Could you check a few things on this drawing? It's one solid part, dimensions in mm from its lowest x, y, z. A direction names the side the tool comes from. Round coordinates to 2 decimals unless told otherwise and drop trailing zeros. Loops run counter-clockwise (first coordinate to the right, second up) from the corner with the lowest first, then second, coordinate; pieces in that order, holes last. Notation, with made-up numbers: M 1,0 L 15,0 A8 ccw 15,7 Z; hole C -0.5,53.25 d1. An arc over 180 degrees is marked long. Return JSON: item names as keys, results as strings.
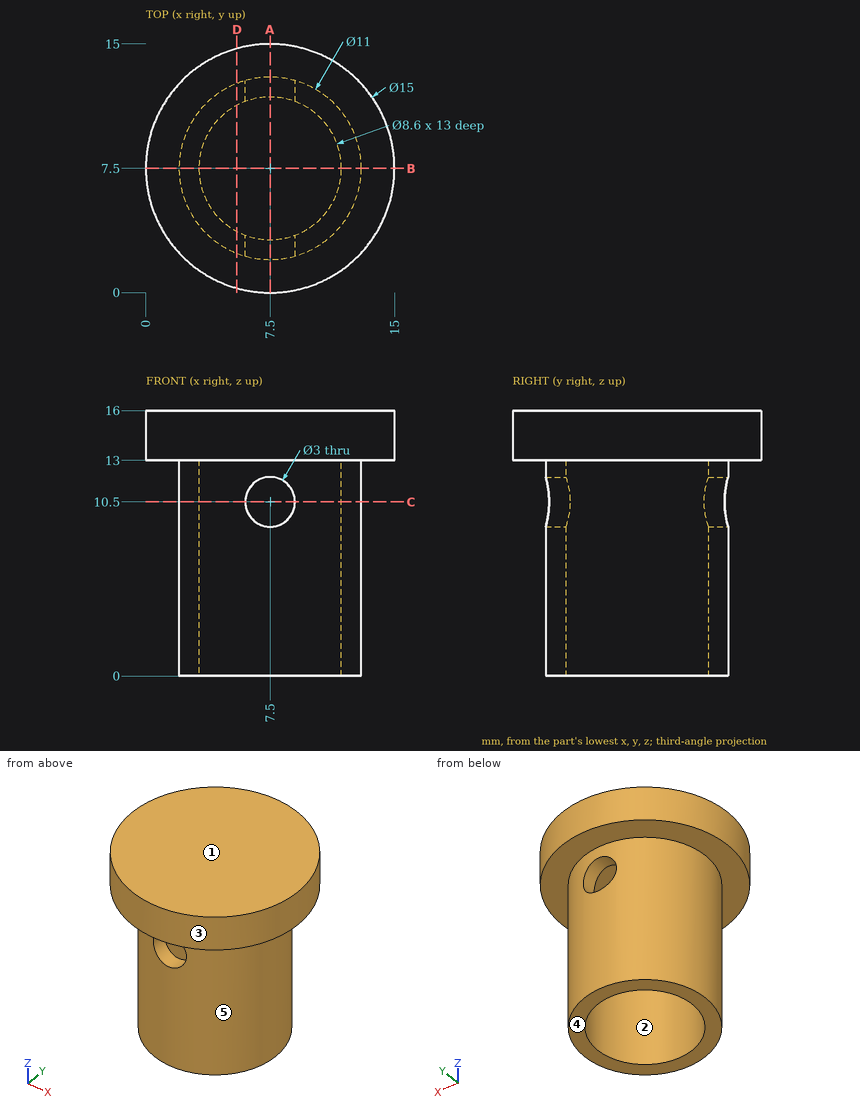
Q1. Suppose I cut it at C-C, the plane z = 10.5. Please give me the cut outline in (x, y), plus the area to 3 significant figures.
Results:
{"outline": "M 6,2.21 L 6,3.47 A4.3 cw 6,11.53 L 6,12.79 A5.5 ccw Z; M 9,2.21 A5.5 ccw 9,12.79 L 9,11.53 A4.3 cw 9,3.47 Z", "area": "29.6 mm2"}
Q2. Suppose I cut it at B-B, the plane y = 7.5. Please give me the cut outline in (x, z).
Results:
{"outline": "M 0,13 L 2,13 L 2,0 L 3.2,0 L 3.2,13 L 11.8,13 L 11.8,0 L 13,0 L 13,13 L 15,13 L 15,16 L 0,16 Z"}
Q3. Suppose I cut it at A-A, the plane x = 7.5. Please give me the cut outline in (y, z), plus the area to 3 significant figures.
Results:
{"outline": "M 0,13 L 2,13 L 2,12 L 3.2,12 L 3.2,13 L 11.8,13 L 11.8,12 L 13,12 L 13,13 L 15,13 L 15,16 L 0,16 Z; M 2,0 L 3.2,0 L 3.2,9 L 2,9 Z; M 11.8,0 L 13,0 L 13,9 L 11.8,9 Z", "area": "69.0 mm2"}
Q4. I'm going to push flat-ended pins straight in: pin 1 Ø4 at (x, z) = (7.5, 10.5) entering from +Y; pin 2 Ø3 at (x, z) = (11.5, 4.5) entering from -Y; pin 3 Ø3 at (y, z) = (11, 8) entering from -X. Where does each tip first touch, or does it pass through?
Results:
{"pin 1": "stops at y = 13", "pin 2": "stops at y = 2.6", "pin 3": "stops at x = 2.38"}
Q5. On a 3-axis mill with a long thin cutter (end or side, diameter ignored), from which of +Z, -Z, +X, -X, +Y, -Y can I reach the whole of each face in a straight line? I mean the marked faces 4 and 5. Say none if no direction works.
Results:
{"face 4": "-Z, +X, -X, +Y, -Y", "face 5": "-Z"}
Q6. Suppose I cut it at D-D, the plane x = 5.5. Please give me the cut outline in (y, z).
Results:
{"outline": "M 0.27,13 L 2.38,13 L 2.38,0 L 3.69,0 L 3.69,13 L 11.31,13 L 11.31,0 L 12.62,0 L 12.62,13 L 14.73,13 L 14.73,16 L 0.27,16 Z"}
Q7. If I drill on line 1 along Y through (x, z) = (7.5, 8.75); line 2 along X through (y, z) = (12.2, 10.5); line 3 along Y through (x, z) = (5.75, 7.5), over which ranges is the centre line in solid material (lowest first)?
Results:
{"line 1": "y = 2 to 3.2, 11.8 to 13", "line 2": "x = 4.64 to 6, 9 to 10.36", "line 3": "y = 2.29 to 3.57, 11.43 to 12.71"}
Q8. Thinking about a two-plate mould opening in X: for the marked faces 1, 2 and 3, which applies, pulls with the +X half, pulls with the -X half, needs draft (parallel to the pull), parting line crosses it, or undercut?
Results:
{"face 1": "needs draft", "face 2": "undercut", "face 3": "parting line crosses it"}
